Verification items for the finished model (mm, model axes). Face numbers are marked on the shaded views. Give positions to 0.01 mm unless a question says otherwise; leave off trailing zeros. Loops run counter-clockwise (first coordinate to the right, second up) from the corner with the lowest first, then second, coordinate; pieces in that order, holes last. Notation, with made-up numbers: M 27,-22 L 32,-22 A25 cw 32,15 Z; hole C -10,22 d1. An arc over 180 degrees is marked long. Answer in a Markdown table with one row per item.
```python
from build123d import *

# Parameters (mm, degrees)
SKETCH1_R           = 30
SKETCH1_R_2         = 6
SKETCH1_R_3         = 1.5
BOSS_EXTRUDE1_DEPTH = 12
CHAMFER1_SIZE       = 1


with BuildPart() as part:
    # Sketch1 → Boss-Extrude1 (new body)
    with BuildSketch(Plane.XY):
        Circle(SKETCH1_R)
        Circle(SKETCH1_R_2, mode=Mode.SUBTRACT)
        with Locations((9, 0)):
            Circle(SKETCH1_R_3, mode=Mode.SUBTRACT)
        with Locations((-4.5, -7.794228634)):
            Circle(SKETCH1_R_3, mode=Mode.SUBTRACT)
        with Locations((-4.5, 7.794228634)):
            Circle(SKETCH1_R_3, mode=Mode.SUBTRACT)
    extrude(amount=BOSS_EXTRUDE1_DEPTH)

    # Chamfer1
    chamfer1_edges = [part.edges().sort_by_distance(p)[0] for p in [
        (-30, 0, 0),
        (-30, 0, 12),
    ]]
    chamfer(chamfer1_edges, length=CHAMFER1_SIZE)


solid = part.part
```
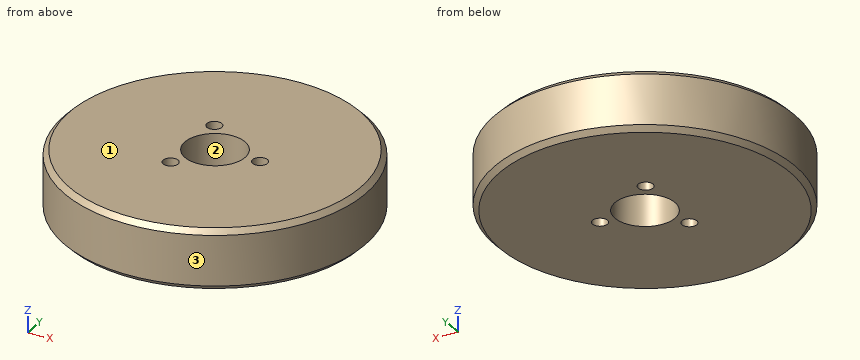
Item 1: Release check for a two-part mould opening along Y. For the marked faces 1, 2 and 3 record: released by +Y, released by -Y, zero draft, split by the parting line, or undercut.
Reported:
| item | result |
|---|---|
| face 1 | zero draft |
| face 2 | undercut |
| face 3 | split by the parting line |
Item 2: Sectioned sample at B-B (y = 0). Record the cut outline in (x, z), and give its area (3 significant figures).
Reported:
| item | result |
|---|---|
| outline | M -30,1 L -29,0 L -6,0 L -6,12 L -29,12 L -30,11 Z; M 6,0 L 7.5,0 L 7.5,12 L 6,12 Z; M 10.5,0 L 29,0 L 30,1 L 30,11 L 29,12 L 10.5,12 Z |
| area | 538 mm^2 |
Item 3: Scan lines: L1, parallel to Y at x = -4.5, z = 5.5; L2, parallel to Y at x = 0, z = 6.5; L3, parallel to X at y = -2, z = 5.5. Record each from-to range of solid material in increasing order. Write a range as [from, to].
Reported:
| item | result |
|---|---|
| L1 | y = [-29.66, -9.29], [-6.29, -3.97], [3.97, 6.29], [9.29, 29.66] |
| L2 | y = [-30, -6], [6, 30] |
| L3 | x = [-29.93, -5.66], [5.66, 29.93] |
Item 4: Go/stop test with flat-tipped pins: pin 1 (2 mm diameter, centred on y = 3.5, z = 9, fed in from -X); pin 2 (6 mm diameter, centred on x = -9.5, z = 6.5, fed in from +Y); pin 3 (3 mm diameter, centred on x = 19, z = 10.5, fed in from -Y). Record where each tip stops, or that it passes through.
Reported:
| item | result |
|---|---|
| pin 1 | stops at x = -29.9 |
| pin 2 | stops at y = 29.29 |
| pin 3 | stops at y = -24.37 |
Item 5: Sectioned sample at C-C (z = 7.75). Record the cut outline in (x, y).
Reported:
| item | result |
|---|---|
| outline | C 0,0 d60; hole C -4.5,-7.79 d3; hole C 0,0 d12; hole C -4.5,7.79 d3; hole C 9,0 d3 |
Item 6: Sectioned sample at A-A (x = 0). Record the cut outline in (y, z), and give its area (3 significant figures).
Reported:
| item | result |
|---|---|
| outline | M -30,1 L -29,0 L -6,0 L -6,12 L -29,12 L -30,11 Z; M 6,0 L 29,0 L 30,1 L 30,11 L 29,12 L 6,12 Z |
| area | 574 mm^2 |
